Autodesk Inventor part; units mm, degrees
ref_plane "YZ Plane" through (0, 0, 0) normal (1, 0, 0) x (0, 1, 0)
ref_plane "XZ Plane" through (0, 0, 0) normal (0, 1, 0) x (-1, 0, 0)
ref_plane "XY Plane" through (0, 0, 0) normal (0, 0, 1) x (1, 0, 0)
sketch "Sketch1" plane through (0, 0, 0) normal (0, 0, 1) x (1, 0, 0)
  line L0 (19.05, -19.05) -> (-19.05, -19.05)
  line L1 (-19.05, -19.05) -> (-19.05, 19.05)
  line L2 (-19.05, 19.05) -> (19.05, 19.05)
  line L3 (19.05, 19.05) -> (19.05, -19.05)
  line L4 (19.05, -19.05) -> (-19.05, 19.05) construction
  line L5 (-19.05, -19.05) -> (19.05, 19.05) construction
  point P0 (0, 0)
  dimension "d0" = 38.1
  dimension "d1" = 38.1
extrude "Extrusion1" add sketch "Sketch1" along normal blind 12.7
sketch "Sketch4" plane through (0, 0, 12.7) normal (0, 0, 1) x (1, 0, 0)
  point P0 (0, 0)
sketch "Sketch5" plane through (0, 0, 12.7) normal (0, 0, 1) x (1, 0, 0)
  line L0 (-19.05, -19.05) -> (19.05, -19.05) construction
  line L1 (19.05, -19.05) -> (19.05, 19.05) construction
  line L2 (19.05, 19.05) -> (-19.05, 19.05) construction
  line L3 (-19.05, 19.05) -> (-19.05, -19.05) construction
  line L4 (15.875, -11.43) -> (-15.875, -11.43) construction
  line L5 (-15.875, -11.43) -> (-15.875, 11.43) construction
  line L6 (-15.875, 11.43) -> (15.875, 11.43) construction
  line L7 (15.875, 11.43) -> (15.875, -11.43) construction
  line L8 (15.875, -11.43) -> (-15.875, 11.43) construction
  line L9 (-15.875, -11.43) -> (15.875, 11.43) construction
  line L10 (11.43, -15.875) -> (-11.43, -15.875) construction
  line L11 (-11.43, -15.875) -> (-11.43, 15.875) construction
  line L12 (-11.43, 15.875) -> (11.43, 15.875) construction
  line L13 (11.43, 15.875) -> (11.43, -15.875) construction
  line L14 (11.43, -15.875) -> (-11.43, 15.875) construction
  line L15 (-11.43, -15.875) -> (11.43, 15.875) construction
  line L16 (0, -8.4414) -> (8.4414, 0) construction
  line L17 (8.4414, 0) -> (0, 8.4414) construction
  line L18 (0, 8.4414) -> (-8.4414, 0) construction
  line L19 (-8.4414, 0) -> (0, -8.4414) construction
  line L20 (-5.969, -5.969) -> (5.969, 5.969) construction
  line L21 (5.969, -5.969) -> (-5.969, 5.969) construction
  line L22 (-8.4414, -8.4414) -> (8.4414, -8.4414) construction
  line L23 (8.4414, -8.4414) -> (8.4414, 8.4414) construction
  line L24 (8.4414, 8.4414) -> (-8.4414, 8.4414) construction
  line L25 (-8.4414, 8.4414) -> (-8.4414, -8.4414) construction
  line L26 (-8.4414, -8.4414) -> (8.4414, 8.4414) construction
  line L27 (8.4414, -8.4414) -> (-8.4414, 8.4414) construction
  point P0 (0, 0)
  point P1 (0, 8.4414)
  point P2 (8.4414, 0)
  point P3 (-15.875, 0)
  point P4 (15.875, 0)
  point P5 (-15.875, 0)
  point P6 (-15.875, 0)
  point P7 (15.875, 0)
  dimension "d46" = 31.75
  dimension "d47" = 22.86
  dimension "d48" = 22.86
  dimension "d49" = 31.75
  dimension "d50" = 11.938
  dimension "d51" = 11.938
  dimension "d52" = 16.8829
  dimension "d53" = 16.8829
  dimension "d54" = 4.445
  dimension "d55" = 7.4336
  dimension "d56" = 5.969
  dimension "d57" = 5.969
  dimension "d58" = 4.445
  dimension "d59" = 7.4336
  dimension "d60" = 9.906
  dimension "d61" = 9.906
  dimension "d62" = 21.844
  dimension "d63" = 21.844
  dimension "d64" = 3.175
  dimension "d65" = 3.175
hole "Hole2" at (-15.875, -11.43, 12.7) at (15.875, -11.43, 12.7) at (15.875, 0, 12.7) at (-15.875, 0, 12.7) at (-15.875, 11.43, 12.7) at (15.875, 11.43, 12.7) direction (0, 0, -1) diameter 3.7973 end through all
sketch "Sketch6" plane through (0, 0, 12.7) normal (0, 0, 1) x (1, 0, 0)
  circle A0 centre (-15.875, 11.43) radius 1.8986 construction
  circle A1 centre (15.875, 0) radius 1.8986 construction
  circle A2 centre (-15.875, -11.43) radius 1.8986 construction
  circle A3 centre (15.875, -11.43) radius 1.8986 construction
  circle A4 centre (-15.875, 0) radius 1.8986 construction
  circle A5 centre (15.875, 11.43) radius 1.8986 construction
  line L0 (-19.05, -19.05) -> (19.05, -19.05) construction
  line L1 (19.05, -19.05) -> (19.05, 19.05) construction
  line L2 (19.05, 19.05) -> (-19.05, 19.05) construction
  line L3 (-19.05, 19.05) -> (-19.05, -19.05) construction
  line L4 (15.875, -11.43) -> (-15.875, -11.43) construction
  line L5 (-15.875, -11.43) -> (-15.875, 11.43) construction
  line L6 (-15.875, 11.43) -> (15.875, 11.43) construction
  line L7 (15.875, 11.43) -> (15.875, -11.43) construction
  line L8 (15.875, -11.43) -> (-15.875, 11.43) construction
  line L9 (-15.875, -11.43) -> (15.875, 11.43) construction
  line L10 (11.43, -15.875) -> (-11.43, -15.875) construction
  line L11 (-11.43, -15.875) -> (-11.43, 15.875) construction
  line L12 (-11.43, 15.875) -> (11.43, 15.875) construction
  line L13 (11.43, 15.875) -> (11.43, -15.875) construction
  line L14 (11.43, -15.875) -> (-11.43, 15.875) construction
  line L15 (-11.43, -15.875) -> (11.43, 15.875) construction
  line L16 (0, -8.4414) -> (8.4414, 0) construction
  line L17 (8.4414, 0) -> (0, 8.4414) construction
  line L18 (0, 8.4414) -> (-8.4414, 0) construction
  line L19 (-8.4414, 0) -> (0, -8.4414) construction
  line L20 (-5.969, -5.969) -> (5.969, 5.969) construction
  line L21 (5.969, -5.969) -> (-5.969, 5.969) construction
  line L22 (-8.4414, -8.4414) -> (8.4414, -8.4414) construction
  line L23 (8.4414, -8.4414) -> (8.4414, 8.4414) construction
  line L24 (8.4414, 8.4414) -> (-8.4414, 8.4414) construction
  line L25 (-8.4414, 8.4414) -> (-8.4414, -8.4414) construction
  line L26 (-8.4414, -8.4414) -> (8.4414, 8.4414) construction
  line L27 (8.4414, -8.4414) -> (-8.4414, 8.4414) construction
  point P0 (0, 0)
  point P1 (0, 8.4414)
  point P2 (8.4414, 0)
  point P3 (8.4414, 0)
  dimension "d73" = 31.75
  dimension "d74" = 22.86
  dimension "d75" = 22.86
  dimension "d76" = 31.75
  dimension "d77" = 11.938
  dimension "d78" = 11.938
  dimension "d79" = 16.8829
  dimension "d80" = 16.8829
  dimension "d81" = 4.445
  dimension "d82" = 7.4336
  dimension "d83" = 5.969
  dimension "d84" = 5.969
  dimension "d85" = 4.445
  dimension "d86" = 7.4336
  dimension "d87" = 9.906
  dimension "d88" = 9.906
  dimension "d89" = 21.844
  dimension "d90" = 21.844
  dimension "d91" = 3.175
  dimension "d92" = 3.175
hole "Hole3" at (-8.4414, 0, 12.7) at (0, 8.4414, 12.7) at (8.4414, 0, 12.7) at (0, -8.4414, 12.7) direction (0, 0, -1) diameter 2.7051 depth 6.35 tip angle 118
properties part number "goniometer_stage_standoff_v1" material "Stainless Steel AISI 304"
Can you work these out from the model? Positions are in its coordinate system, mm. A direction names the side the tool comes from. Give positions to 0.01 mm unless a question says otherwise; leave off trailing zeros. Write each loop counter-clockwise with the first axis right and the second up, starting at its lowest first coordinate (ties: lowest second). Pieces come first, ordered by that corner, then holes. Notation, with made-up numbers: M 16.5,41.25 L 41.5,41.25 A22 ccw 41.5,78.25 Z; hole C 54,89.5 d7. An arc over 180 degrees is marked long. Answer in a Markdown table with one row per item. Add a question column.
Item 1: On a 3-axis mill with a long thin cutter (end or side, diameter ignored), from which of +Z, -Z, +X, -X, +Y, -Y can I reach the whole of each face in a straight line? I mean faces 5 (the cylindrical face through (-17.476, -1.021, 6.261)), 6 (the cylindrical face through (0.5, -9.7, 9.5)). Say none if no direction works.
Item 2: Please list where these lines run through material, in increasing order: L1, parallel to X at y = -11.43, z = 4.5; L2, parallel to X at y = 0, z = 7.25; L3, parallel to Y at x = 17, z = 5.
Item 3: We'd pull the mould along Y, two halves only. Please class faces 1 (the flat face through (0, 19.05, 6)), 2 (the conical face through (0.01, -8.207, 5.678)), 3 (the flat face through (0, -19.05, 6)), 4 (the cylindrical face through (13.993, -11.183, 6.261)): released by +Y, released by -Y, zero draft, split by the parting line, or undercut.
Item 4: Imagine slicing it at B-B, the plane z = 7.25. State how many separate pieces and enclosed holes the cut face has, plus the area to 3 significant figures.
Item 5: Imagine slicing it at A-A, the plane y = 11.43. Write out the boundary of the cut face in (x, z).
Item 6: Imagine slicing it at C-C, the plane z = 3. Write out the boundary of the cut face in (x, y) (3 decimals), plus the area to 3 significant figures.
Item 7: For pin 1 Ø3.5 at (x, y) = (-15.875, -11.43) entering from -Z; pin 2 Ø1.6 at (x, y) = (-8.44, 0) entering from +Z, each with a flat end and sliding along its axis, tell me the tip position at first contact or that it passes through.
Evaluation:
| question | item | result |
|---|---|---|
| 1 | face 5 | +Z, -Z |
| 1 | face 6 | +Z |
| 2 | L1 | x = -19.05 to -17.77, -13.98 to 13.98, 17.77 to 19.05 |
| 2 | L2 | x = -19.05 to -17.77, -13.98 to -9.79, -7.09 to 7.09, 9.79 to 13.98, 17.77 to 19.05 |
| 2 | L3 | y = -19.05 to -12.96, -9.9 to -1.53, 1.53 to 9.9, 12.96 to 19.05 |
| 3 | face 1 | released by +Y |
| 3 | face 2 | undercut |
| 3 | face 3 | released by -Y |
| 3 | face 4 | undercut |
| 4 | separate pieces | 1 |
| 4 | enclosed holes | 10 |
| 4 | area | 1,360 mm² |
| 5 | outline | M -19.05,0 L -17.77,0 L -17.77,12.7 L -19.05,12.7 Z; M -13.98,0 L 13.98,0 L 13.98,12.7 L -13.98,12.7 Z; M 17.77,0 L 19.05,0 L 19.05,12.7 L 17.77,12.7 Z |
| 6 | outline | M -19.05,-19.05 L 19.05,-19.05 L 19.05,19.05 L -19.05,19.05 Z; hole C -15.875,-11.43 d3.797; hole C -15.875,0 d3.797; hole C -15.875,11.43 d3.797; hole C 15.875,-11.43 d3.797; hole C 15.875,0 d3.797; hole C 15.875,11.43 d3.797 |
| 6 | area | 1,380 mm² |
| 7 | pin 1 | passes through |
| 7 | pin 2 | stops at z = 6.02 |
